The listing builds one solid part. Answer for the finished solid, in the listing's coordinates (mm). A direction names the side the tool comes from. Round coordinates to 2 decimals unless told otherwise and drop trailing zeros. Loops run counter-clockwise (first coordinate to the right, second up) from the corner with the lowest first, then second, coordinate; pieces in that order, holes last. Notation, with made-up numbers: (-14.75, 73) -> (10.25, 73) arc R29 cw to (10.25, 102) -> close; hole circle Ø7 at (62, -33.5). An arc over 180 degrees is marked (long way). Use a Markdown table: item, result. Add a question column.
Q1. Consider line 1 (Z direction, x = 42, y = -1.75); line 2 (Y direction, x = 145, z = -4.25). Determine where each line is inside the solid, lowest interval first.
Q2. Which of the six approach directions +Z, -Z, +X, -X, +Y, -Y give full straight-line access (tool end or side, diameter ignored) to faces 1 (the flat face through (136, -4, 0)), 2 (the flat face through (136, -5, 0))?
Q3. Section A-A on x = 60.5 is taken. Give the vertices of the cut face in (y, z).
Q4. Given pin 1 Ø3.5 at (x, y) = (145, 0) entering from +Z; pin 2 Ø2.5 at (x, y) = (5, 0) entering from +Z, each flat-ended and moving along its own axis, determine where each tip first touches the part or whether it passes through.
Q5. For a pull along Z with two mould halves and no side action, classify faces 3 (the flat face through (0, -4.5, 0.1)), 4 (the flat face through (136, 0, 4)), 5 (the flat face through (136, 0, -5)) as released by +Z, released by -Z, zero draft, split by the parting line, or undercut.
from build123d import *

# Parameters (mm, degrees)
F0_W     = 10
F0_H     = 10
F0_W_2   = 8
F0_H_2   = 8
F1_DEPTH = 275
F2_R     = 1.5
F3_DEPTH = 25
F4_R     = 2
F4_R_2   = 1.5
F5_DEPTH = 25


with BuildPart() as f1:
    # F0 (on Right) → F1 (new body)
    with BuildSketch(Plane.YZ):
        Rectangle(F0_W, F0_H)
        Rectangle(F0_W_2, F0_H_2, mode=Mode.SUBTRACT)
    extrude(amount=F1_DEPTH)

    # F2 (on face) → F3 (cut)
    with BuildSketch(Plane.XY.offset(5)):
        with Locations((130, 0)):
            Circle(F2_R)
        with Locations((5, 0)):
            Circle(F2_R)
        with Locations((145, 0)):
            Circle(F2_R)
        with Locations((270, 0)):
            Circle(F2_R)
    extrude(amount=-F3_DEPTH, mode=Mode.SUBTRACT)

    # F4 (on face) → F5 (cut)
    with BuildSketch(Plane(origin=(0, 5, 0), x_dir=(-1, 0, 0), z_dir=(0, 1, 0))):
        with Locations((-233.5, 0)):
            Circle(F4_R)
        with Locations((-195.5, 0)):
            Circle(F4_R)
        with Locations((-79.5, 0)):
            Circle(F4_R)
        with Locations((-41.5, 0)):
            Circle(F4_R)
        with Locations((-260, 0)):
            Circle(F4_R_2)
        with Locations((-15, 0)):
            Circle(F4_R_2)
    extrude(amount=-F5_DEPTH, mode=Mode.SUBTRACT)


solid = f1.part
Checked values:
| question | item | result |
|---|---|---|
| 1 | line 1 | z = -5 to -4, 4 to 5 |
| 1 | line 2 | y = -5 to -1.5, 1.5 to 5 |
| 2 | face 1 | +X, -X |
| 2 | face 2 | +Z, -Z, +X, -X, -Y |
| 3 | outline | (-5, -5) -> (5, -5) -> (5, 5) -> (-5, 5) -> close; hole (-4, -4) -> (4, -4) -> (4, 4) -> (-4, 4) -> close |
| 4 | pin 1 | stops at z = 5 |
| 4 | pin 2 | passes through |
| 5 | face 3 | zero draft |
| 5 | face 4 | undercut |
| 5 | face 5 | released by -Z |
